Could you check a few things on this model? Use its own coordinates, in mm. A direction names the side the tool comes from. Round coordinates to 2 decimals unless told otherwise and drop trailing zeros. Write each loop counter-clockwise with the first axis right and the second up, starting at its lowest first coordinate (ties: lowest second). Pieces come first, ordered by that corner, then holes. Notation, with made-up numbers: (-10.75, 25) -> (9.25, 25) arc R37 ccw to (9.25, 61) -> close; hole circle Ø6 at (58.5, 86.5). An arc over 180 degrees is marked (long way). One line per question, with ' | ' between items. Start each with the question number.
1. Imagine slicing it at B-B, the plane z = -6. List the corners of the cut face in (x, y) for me.
2. Imagine slicing it at A-A, the plane y = 44. List the corners of the cut face in (x, z) for me.
3. For faces 5 (the flat face through (6, 25, 12)), 6 (the flat face through (0, 25, -14)), which set-ups out of +Z, -Z, +X, -X, +Y, -Y let a thin tool reach every point of the face, with its end or its side?
4. Imagine slicing it at D-D, the plane z = -22.5. List the corners of the cut face in (x, y) for me, and give its area (3 significant figures).
5. For pin 1 Ø14 at (y, z) = (20.5, -9.5) entering from +X; pin 2 Ø3 at (y, z) = (44, -6) entering from -X; pin 3 Ø1.6 at (x, y) = (1, 25) entering from -Z; pin 4 Ø8 at (x, y) = (8, 15) entering from -Z, each with a flat end and sliding along its axis, tell me the tip position at first contact or that it passes through.
6. If I drill on line 1 along Y through (x, z) = (-4.25, -6); line 2 along Y through (x, z) = (-4, -21.5); line 3 along X through (y, z) = (40, -18.5), over which ranges is the centre line in solid material (lowest first)? Write a range as [from, to].
7. Imagine slicing it at C-C, the plane y = 10. List the corners of the cut face in (x, z) for me, and give its area (3 significant figures).
8. Thinking about a two-plate mould opening in Y: for faces 1 (the cylindrical face through (-4.06, 45.24, -22.16)), 2 (the flat face through (-0.4, 50, -3.8)), 3 (the cylindrical face through (-4.056, 4.891, -21.423)), 4 (the flat face through (-8, 25, -8)), which applies, released by +Y, released by -Y, zero draft, split by the parting line, or undercut?
from build123d import *

# Parameters (mm, degrees)
EXTRUDE_1_DEPTH    = 50
HOLE_WIZARD_M3_1_D = 2.5


with BuildPart() as part:
    # 草图1 → 凸台-拉伸1 (new body)
    with BuildSketch(Plane(origin=(0, 0, 0), x_dir=(1, 0, 0), z_dir=(0, 1, 0))):
        with BuildLine():
            Line((0, 0), (0, 28))
            Line((0, 28), (-8, 28))
            Line((-8, 28), (-8, -12))
            Line((-8, -12), (20, -12))
            Line((20, -12), (20, 0))
            Line((20, 0), (18, 0))
            ThreePointArc((18, 0), (10, -8), (2, 0))
            Line((2, 0), (0, 0))
        make_face()
    extrude(amount=EXTRUDE_1_DEPTH)

    # M3 螺纹孔1 (through all)
    with Locations(Plane(origin=(0, 0, 0), x_dir=(0, 0, -1), z_dir=(1, 0, 0))):
        with Locations((22, 44), (6, 44), (6, 6), (22, 6)):
            Hole(HOLE_WIZARD_M3_1_D / 2)


solid = part.part
Geometry results:
1) outline: (-8, 0) -> (0, 0) -> (0, 4.75) -> (-8, 4.75) -> close; (-8, 7.25) -> (0, 7.25) -> (0, 42.75) -> (-8, 42.75) -> close; (-8, 45.25) -> (0, 45.25) -> (0, 50) -> (-8, 50) -> close
2) outline: (-8, -28) -> (0, -28) -> (0, -23.25) -> (-8, -23.25) -> close; (-8, -20.75) -> (0, -20.75) -> (0, -7.25) -> (-8, -7.25) -> close; (-8, -4.75) -> (0, -4.75) -> (0, 0) -> (2, 0) arc R8 cw to (18, 0) -> (20, 0) -> (20, 12) -> (-8, 12) -> close
3) face 5: +Z, +X, -X, +Y, -Y | face 6: -Z, +X, +Y, -Y
4) outline: (-8, 0) -> (0, 0) -> (0, 4.85) -> (-8, 4.85) -> close; (-8, 7.15) -> (0, 7.15) -> (0, 42.85) -> (-8, 42.85) -> close; (-8, 45.15) -> (0, 45.15) -> (0, 50) -> (-8, 50) -> close | area: 363 mm2
5) pin 1: stops at x = 0 | pin 2: stops at x = -8 | pin 3: stops at z = 0 | pin 4: stops at z = 5.29
6) line 1: y = [0, 4.75], [7.25, 42.75], [45.25, 50] | line 2: y = [0, 4.85], [7.15, 42.85], [45.15, 50] | line 3: x = [-8, 0]
7) outline: (-8, -28) -> (0, -28) -> (0, 0) -> (2, 0) arc R8 cw to (18, 0) -> (20, 0) -> (20, 12) -> (-8, 12) -> close | area: 459 mm2
8) face 1: undercut | face 2: released by +Y | face 3: undercut | face 4: zero draft
